Design review of the part built by this model. Coordinates are the model's own, in mm. A direction names the side the tool comes from. Coordinates: 2 decimals unless noted, no trailing zeros. Order: outer loops, then holes, each group sorted by start corner. A loop starts at its lowest first (then second) coordinate and runs counter-clockwise, first axis right, second up. Notation, with made-up numbers: (-34, 4.5) -> (-3, 4.5) arc R20 cw to (-3, 39.5) -> close; hole circle Ø7 at (-7, 25). An arc over 180 degrees is marked (long way). Use a Markdown table: item, result. Add a question column.
Q1. Insertion check: pin 1 (12 mm diameter, centred on x = 3.5, y = 53, fed in from -Z); pin 2 (15 mm diameter, centred on y = 25, z = 0, fed in from +X); pin 3 (8 mm diameter, centred on y = 25, z = 0, fed in from -X); pin 4 (2 mm diameter, centred on y = 180.5, z = 17.5, fed in from -X). Each pin has a flat end and moves straight along its axis. Give the tip position at first contact, or say it passes through.
Q2. Add section C-C (y = 37). State the section outline as (x, z) points.
Q3. The part is to be moulded in two halves that separate along Z. For faces 1 (the face through (-25, 25, 0)), 2 (the face through (-34.1, 25.37, 8.49)), 3 (the face through (-45, 20, -4.4)), say which applies: pulls with the +Z half, pulls with the -Z half, needs draft (parallel to the pull), parting line crosses it, or undercut.
Q4. Machinability: for faces 4 (the face through (-34.424, 31.445, 0.846)), 5 (the face through (45, 20, -4.4)), 6 (the face through (-22, 25, 0)), 7 (the face through (34.1, 25.37, 8.49)), 8 (the face through (1.7, 0, 22.1)), which of the approach directions +Z, -Z, +X, -X, +Y, -Y give a long, thin tool a straight path to every point of the face, cutting with its end or side? Answer none if there is none.
Q5. Add section B-B (x = 3). State the section outline as (y, z) points, then the cut area to 3 significant figures.
Q6. Wall thickness on probe 1 along Z at (x, y) = (-11, 25); probe 2 along X at (y, z) = (173, 1); probe 3 along Y at (x, z) = (-12, 0): over which ranges is each line inside the solid? List them lowest first.
Q7. Add section D-D (x = 39). State the section outline as (y, z) points.
from build123d import *

# Parameters (mm, degrees)
SKETCH2_R                = 25
SKETCH2_R_2              = 22
BOSS_EXTRUDE1_DEPTH      = 250
SKETCH3_R                = 8.5
SKETCH3_R_2              = 6.5
BOSS_EXTRUDE2_DEPTH      = 45
BOSS_EXTRUDE2_DEPTH_BACK = 45


with BuildPart() as part:
    # Sketch2 → Boss-Extrude1 (new body)
    with BuildSketch(Plane(origin=(0, 0, 0), x_dir=(1, 0, 0), z_dir=(0, 1, 0))):
        Circle(SKETCH2_R)
        Circle(SKETCH2_R_2, mode=Mode.SUBTRACT)
    extrude(amount=BOSS_EXTRUDE1_DEPTH)

    # Sketch3 → Boss-Extrude2 (add, two sides)
    with BuildSketch(Plane(origin=(0, 0, 0), x_dir=(0, 0, -1), z_dir=(1, 0, 0))) as boss_extrude2_sk:
        with Locations((0, 25)):
            Circle(SKETCH3_R)
        with Locations((0, 25)):
            Circle(SKETCH3_R_2, mode=Mode.SUBTRACT)
    extrude(amount=BOSS_EXTRUDE2_DEPTH)
    extrude(boss_extrude2_sk.sketch, amount=-BOSS_EXTRUDE2_DEPTH_BACK)


solid = part.part
Established:
| question | item | result |
|---|---|---|
| 1 | pin 1 | z = -25 |
| 1 | pin 2 | x = 45 |
| 1 | pin 3 | x = -25 |
| 1 | pin 4 | x = -18.78 |
| 2 | outline | circle Ø50 at (0, 0); hole circle Ø44 at (0, 0) |
| 3 | face 1 | undercut |
| 3 | face 2 | parting line crosses it |
| 3 | face 3 | needs draft |
| 4 | face 4 | -X |
| 4 | face 5 | +Z, -Z, +X, +Y, -Y |
| 4 | face 6 | none |
| 4 | face 7 | +X |
| 4 | face 8 | +Z, -Z, +X, -X, -Y |
| 5 | outline | (0, -24.82) -> (250, -24.82) -> (250, -21.79) -> (0, -21.79) -> close; (0, 21.79) -> (250, 21.79) -> (250, 24.82) -> (0, 24.82) -> close; circle Ø17 at (25, 0); hole circle Ø13 at (25, 0) |
| 5 | area | 1,610 mm^2 |
| 6 | probe 1 | -22.45 to -19.05, -8.5 to -6.5, 6.5 to 8.5, 19.05 to 22.45 |
| 6 | probe 2 | -24.98 to -21.98, 21.98 to 24.98 |
| 6 | probe 3 | 16.5 to 18.5, 31.5 to 33.5 |
| 7 | outline | circle Ø17 at (25, 0); hole circle Ø13 at (25, 0) |
